Design review of the part shown in the three views and the two pictorial views. Dimensions are in mm from the part's minimum x, y and z. A direction names the side the tool comes from. Give positions to 0.01 mm unless a question says otherwise; leave off trailing zeros. Loops run counter-clockwise (first coordinate to the right, second up) from the corner with the lowest first, then second, coordinate; pieces in that order, holes last.
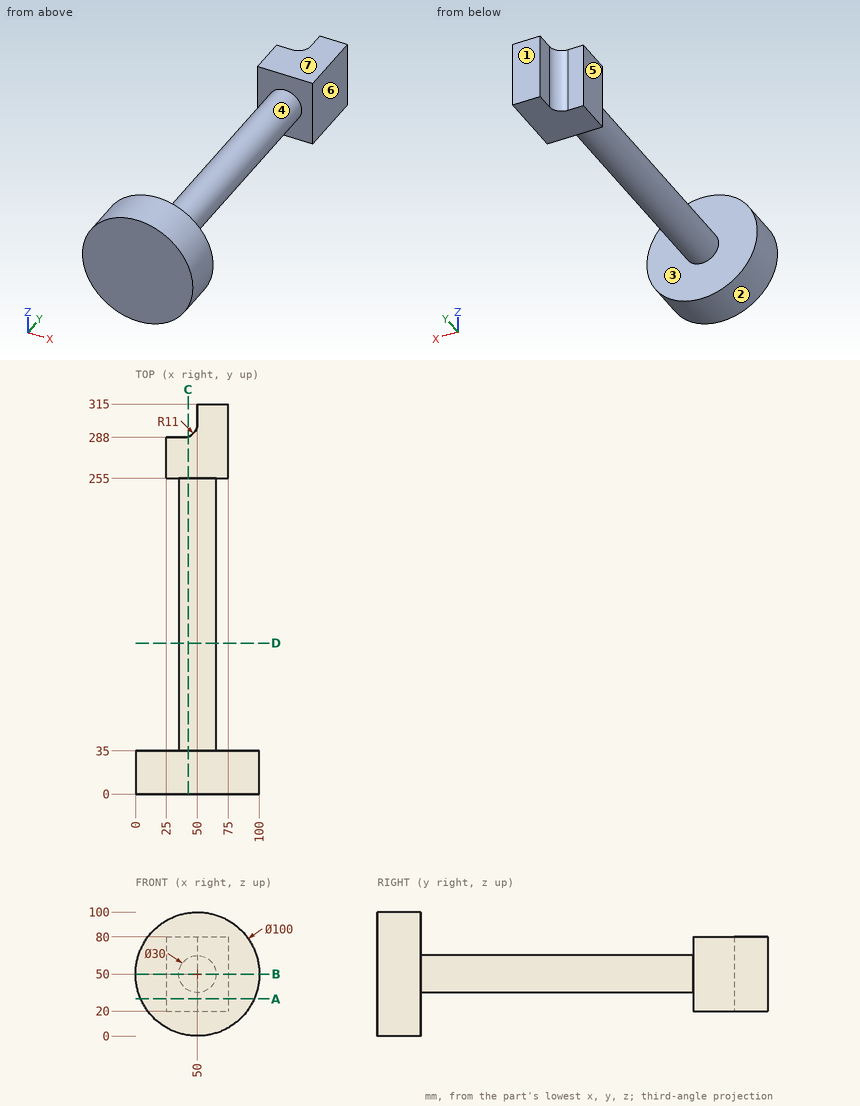
Q1. Consider section B-B on z = 50. Give the boundary of the cut face in (x, y), plus the area to 3 significant figures.
Answers:
outline: (0, 0) - (100, 0) - (100, 35) - (65, 35) - (65, 255) - (75, 255) - (75, 315) - (50, 315) - (50, 299) arc R11 cw to (39, 288) - (25, 288) - (25, 255) - (35, 255) - (35, 35) - (0, 35) - close
area: 12,500 mm2
Q2. For pin 1 Ø10 at (x, y) = (58.5, 228.5) entering from -Z; pin 2 Ø15 at (x, y) = (61.5, 286) entering from +Z; pin 3 Ø5 at (y, z) = (308.5, 41) entering from -X, all flat-tipped, find the tip position at first contact; note any pin that passes through.
Answers:
pin 1: stops at z = 35.41
pin 2: stops at z = 80
pin 3: stops at x = 50
Q3. Mouldability with a two-part tool opening along Y and no side actions: class the marked faces 1, 2 and 3 as +Y half, -Y half, draft (parallel to the pull), parting line (faces both ways), or undercut.
Answers:
face 1: +Y half
face 2: draft
face 3: undercut
Q4. Machinability: for the marked faces 4, 5, 6 and 7, which of the approach directions +Z, -Z, +X, -X, +Y, -Y give a long, thin tool a straight path to every point of the face, cutting with its end or side? Answer none if there is none.
Answers:
face 4: none
face 5: +Z, -Z, -X, +Y
face 6: +Z, -Z, +X, +Y
face 7: +Z, +X, -X, +Y
Q5. Consider section D-D on y = 122. Give the boundary of the cut face in (x, z).
Answers:
outline: circle Ø30 at (50, 50)
Q6. Consider section C-C on x = 42.5. Give the boundary of the cut face in (y, z).
Answers:
outline: (0, 0.57) - (35, 0.57) - (35, 37.01) - (255, 37.01) - (255, 20) - (288.57, 20) - (288.57, 80) - (255, 80) - (255, 62.99) - (35, 62.99) - (35, 99.43) - (0, 99.43) - close
Q7. Consider section A-A on z = 30. Give the boundary of the cut face in (x, y), plus the area to 3 significant figures.
Answers:
outline: (4.17, 0) - (95.83, 0) - (95.83, 35) - (4.17, 35) - close; (25, 255) - (75, 255) - (75, 315) - (50, 315) - (50, 299) arc R11 cw to (39, 288) - (25, 288) - close
area: 5,560 mm2
Q8. For probe 1 along Y at (x, z) = (38, 30); probe 2 along Y at (x, z) = (69, 39); probe 3 along Z at (x, y) = (49, 73), list the stretches that pass through material, from the lowest coordinate up.
Answers:
probe 1: y = 0 to 35, 255 to 288
probe 2: y = 0 to 35, 255 to 315
probe 3: z = 35.03 to 64.97
